```python
from build123d import *

# Parameters (mm, degrees)
SKETCH1_W           = 60
SKETCH1_H           = 25.25
BOSS_EXTRUDE1_DEPTH = 1.5875
SKETCH2_W           = 42
SKETCH2_H           = 3.18
SKETCH2_W_2         = 5.7
SKETCH2_W_3         = 5.8
CUT_EXTRUDE1_DEPTH  = 1.5875


with BuildPart() as part:
    # Sketch1 → Boss-Extrude1 (new body)
    with BuildSketch(Plane.XY):
        with Locations((0, 12.625)):
            Rectangle(SKETCH1_W, SKETCH1_H)
    boss_extrude1 = extrude(amount=BOSS_EXTRUDE1_DEPTH)

    # Sketch2 → Cut-Extrude1 (cut)
    with BuildSketch(Plane.XY.offset(1.5875)):
        with Locations((0, 23.66)):
            Rectangle(SKETCH2_W, SKETCH2_H)
        with Locations((29.85, 23.66)):
            Rectangle(SKETCH2_W_2, SKETCH2_H)
        with Locations((-29.9, 23.66)):
            Rectangle(SKETCH2_W_3, SKETCH2_H)
    cut_extrude1 = extrude(amount=-CUT_EXTRUDE1_DEPTH, mode=Mode.SUBTRACT)

    # Mirror1: Boss-Extrude1, Cut-Extrude1 across plane
    add(boss_extrude1.mirror(Plane.ZX))
    add(cut_extrude1.mirror(Plane.ZX), mode=Mode.SUBTRACT)


solid = part.part
```
For this review, take the finished solid that the model builds, in its own axes (mm). A direction names the side the tool comes from. Give positions to 0.01 mm unless a question says otherwise; leave off trailing zeros. Write each loop counter-clockwise with the first axis right and the second up, starting at its lowest first coordinate (ties: lowest second). Pieces come first, ordered by that corner, then holes. Notation, with made-up numbers: M 35.5,79 L 80.5,79 A30 cw 80.5,118 Z; hole C 49,73 d9. An arc over 180 degrees is marked long. Answer as CSV lines item,"result".
1. For faces 1 (the flat face through (-21, 24, 1)), 2 (the flat face through (21, -24, 1)), 3 (the flat face through (28, -22.07, 1)), list the 3-axis set-ups (+Z, -Z, +X, -X, +Y, -Y) from which the entire face can be reached by the end or side of a thin tool; tool diameter is ignored.
Findings:
face 1,"+Z, -Z, +Y"
face 2,"+Z, -Z, -Y"
face 3,"+Z, -Z, +X, -Y"
2. Consider section B-B, the plane x = 7. Write out the cut boundary in (y, z).
Findings:
outline,"M -22.07,0 L 22.07,0 L 22.07,1.59 L -22.07,1.59 Z"
3. Consider section A-A, the plane z = 0.4. Write out the cut boundary in (x, y), then the cut area to 3 significant figures.
Findings:
outline,"M -30,-22.07 L -27,-22.07 L -27,-25.25 L -21,-25.25 L -21,-22.07 L 21,-22.07 L 21,-25.25 L 27,-25.25 L 27,-22.07 L 30,-22.07 L 30,22.07 L 27,22.07 L 27,25.25 L 21,25.25 L 21,22.07 L -21,22.07 L -21,25.25 L -27,25.25 L -27,22.07 L -30,22.07 Z"
area,"2,720 mm2"
4. Draft analysis for pull direction X (two halves, no side actions). For faces 4 (the flat face through (0, 0, 0)), 5 (the flat face through (0, 22.07, 1)), 6 (the flat face through (27, 24, 1)), state which applies: +X half, -X half, draft (parallel to the pull), parting line (faces both ways), or undercut.
Findings:
face 4,"draft"
face 5,"undercut"
face 6,"+X half"
5. Wall thickness on line 1 (Y direction, x = -13.5, z = 1.4): over which ranges is the line inside the solid? List them lowest first.
Findings:
line 1,"y = -22.07 to 22.07"
6. For pin 1 (0.8 mm diameter, centred on x = -29, z = 0.5, fed in from +Y); pin 2 (0.5 mm diameter, centred on y = 24, z = 0.5, fed in from +X); pin 3 (0.5 mm diameter, centred on x = -2, z = 0.5, fed in from -Y), all flat-tipped, find the tip position at first contact; note any pin that passes through.
Findings:
pin 1,"stops at y = 22.07"
pin 2,"stops at x = 27"
pin 3,"stops at y = -22.07"
